Input: part model. Units: mm. Frame: model coordinates. Give positions to 0.01 mm unless a question says otherwise; leave off trailing zeros. Loops run counter-clockwise (first coordinate to the right, second up) from the corner with the lowest first, then second, coordinate; pieces in that order, holes last. Notation, with made-up numbers: (32, 71.5) -> (64, 71.5) arc R8 cw to (64, 83.5) -> close; hole circle Ø8 at (27, 12.5). An arc over 180 degrees is marked (long way). Answer as a JSON object with one key per item and string values. Group by question number.
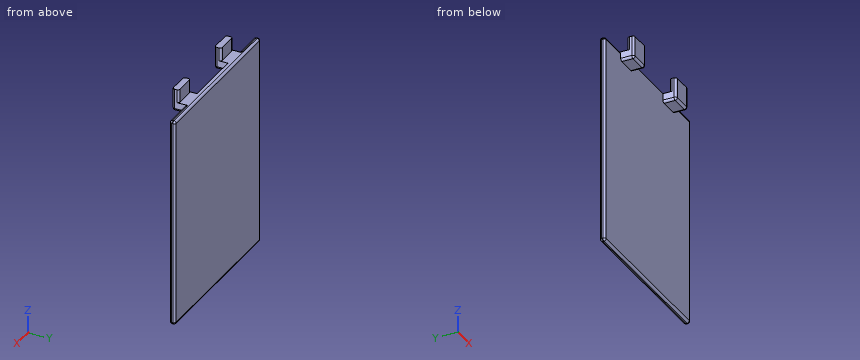
Autodesk Inventor part; units mm, degrees
ref_plane "YZ Plane" through (0, 0, 0) normal (1, 0, 0) x (0, 1, 0)
ref_plane "XZ Plane" through (0, 0, 0) normal (0, 1, 0) x (-1, 0, 0)
ref_plane "XY Plane" through (0, 0, 0) normal (0, 0, 1) x (1, 0, 0)
sketch "Sketch1" plane through (0, 0, 0) normal (0, 1, 0) x (-1, 0, 0)
  line L0 (36.4, 47.4) -> (-36.4, 47.4)
  line L1 (-37.4, 46.4) -> (-37.4, -46.4)
  line L2 (-36.4, -47.4) -> (36.4, -47.4)
  line L3 (37.4, -46.4) -> (37.4, 46.4)
  line L4 (37.4, 47.4) -> (-37.4, -47.4) construction
  line L5 (-37.4, 47.4) -> (37.4, -47.4) construction
  arc A0 (37.4, 46.4) -> (36.4, 47.4) centre (36.4, 46.4) ccw
  arc A1 (-36.4, 47.4) -> (-37.4, 46.4) centre (-36.4, 46.4) ccw
  arc A2 (-37.4, -46.4) -> (-36.4, -47.4) centre (-36.4, -46.4) ccw
  arc A3 (36.4, -47.4) -> (37.4, -46.4) centre (36.4, -46.4) ccw
  point P0 (0, 0)
  dimension "d0" = 94.8
  dimension "d1" = 74.8
  dimension "d2" = 1
extrude "Extrusion1" add sketch "Sketch1" along normal blind 2.5
sketch "Sketch2" plane through (0, 0, 0) normal (0, -1, 0) x (1, 0, 0)
  line L0 (0, 0) -> (-37.4, 0)
  line L1 (-37.4, 0) -> (-37.4, 47.4)
  line L2 (-37.4, 47.4) -> (0, 47.4)
  line L3 (0, 47.4) -> (0, 0)
  line L4 (-23.7, 51.4) -> (-13.7, 51.4)
  line L5 (-13.7, 51.4) -> (-13.7, 43.4)
  line L6 (-13.7, 43.4) -> (-23.7, 43.4)
  line L7 (-23.7, 43.4) -> (-23.7, 51.4)
  line L8 (-36.4, 47.4) -> (36.4, 47.4)
  line L9 (-23.7, 51.4) -> (-13.7, 43.4) construction
  line L10 (-13.7, 51.4) -> (-23.7, 43.4) construction
  line L11 (0, 0) -> (36.5961, 0)
  line L12 (36.5961, 0) -> (36.5961, 47.4)
  line L13 (36.5961, 47.4) -> (0, 47.4)
  line L14 (0, 47.4) -> (0, 0)
  line L15 (13.2981, 51.4) -> (23.2981, 51.4)
  line L16 (23.2981, 51.4) -> (23.2981, 43.4)
  line L17 (23.2981, 43.4) -> (13.2981, 43.4)
  line L18 (13.2981, 43.4) -> (13.2981, 51.4)
  line L19 (13.2981, 51.4) -> (23.2981, 43.4) construction
  line L20 (23.2981, 51.4) -> (13.2981, 43.4) construction
  point P0 (-18.7, 47.4)
  point P1 (18.2981, 47.4)
  point P2 (23.2981, 47.4)
  point P3 (13.2981, 47.4)
  point P4 (-13.7, 47.4)
  point P5 (-23.7, 47.4)
  dimension "d5" = 10
  dimension "d6" = 8
  dimension "d7" = 10
  dimension "d8" = 8
extrude "Extrusion2" add sketch "Sketch2" along normal blind 6 contours L5 L6 L7 L2 | L8 L16 L17 L18
sketch "Sketch3" plane through (-36.4, 2.5, 47.4) normal (0, 0, 1) x (1, 0, 0)
  line L0 (12.7, -8.5) -> (22.7, -8.5)
  line L1 (22.7, -2.5) -> (22.7, -8.5)
  line L2 (13.7, -8.5) -> (21.7, -8.5)
  line L3 (22.7, -7.5) -> (22.7, -6.5)
  line L4 (21.7, -5.5) -> (13.7, -5.5)
  line L5 (12.7, -6.5) -> (12.7, -7.5)
  line L6 (59.6981, -2.5) -> (59.6981, -8.5)
  line L7 (50.6981, -8.5) -> (58.6981, -8.5)
  line L8 (59.6981, -7.5) -> (59.6981, -6.5)
  line L9 (58.6981, -5.5) -> (50.6981, -5.5)
  line L10 (49.6981, -6.5) -> (49.6981, -7.5)
  arc A0 (13.7, -5.5) -> (12.7, -6.5) centre (13.7, -6.5) ccw
  arc A1 (22.7, -6.5) -> (21.7, -5.5) centre (21.7, -6.5) ccw
  arc A2 (21.7, -8.5) -> (22.7, -7.5) centre (21.7, -7.5) ccw
  arc A3 (12.7, -7.5) -> (13.7, -8.5) centre (13.7, -7.5) ccw
  arc A4 (50.6981, -5.5) -> (49.6981, -6.5) centre (50.6981, -6.5) ccw
  arc A5 (59.6981, -6.5) -> (58.6981, -5.5) centre (58.6981, -6.5) ccw
  arc A6 (58.6981, -8.5) -> (59.6981, -7.5) centre (58.6981, -7.5) ccw
  arc A7 (49.6981, -7.5) -> (50.6981, -8.5) centre (50.6981, -7.5) ccw
  line L11 (49.0159, -7.1882) -> (60.5232, -7.1882)
  line L12 (60.5232, -7.1882) -> (60.5232, -9.9786)
  line L13 (60.5232, -9.9786) -> (49.0159, -9.9786)
  line L14 (49.0159, -9.9786) -> (49.0159, -7.1882)
  line L15 (11.7436, -7.1882) -> (24.9599, -7.1882)
  line L16 (24.9599, -7.1882) -> (24.9599, -11.0237)
  line L17 (24.9599, -11.0237) -> (11.7436, -11.0237)
  line L18 (11.7436, -11.0237) -> (11.7436, -7.1882)
  line L19 (49.6981, -8.5) -> (59.6981, -8.5)
  line L20 (49.0159, -8.5834) -> (59.6981, -8.5)
  line L21 (49.6981, -8.5) -> (59.6981, -8.5)
  point P0 (36.4, -2.5)
  point P1 (22.7, -5.5)
  point P2 (59.6981, -5.5)
  point P3 (12.7, -7.1882)
  point P4 (22.7, -7.1882)
  point P5 (49.6981, -7.1882)
  dimension "d11" = 1
extrude "Extrusion3" add sketch "Sketch3" along normal blind 6 contours A3 L5 L15 L1 A2 L0 | L5 A0 L4 A1 L1 L15 | A6 L7 A7 L10 L11 L6 | L11 L10 A4 L9 A5 L6
extrude "Extrusion4" cut sketch "Sketch3" against normal blind 6 contours L0 L1 L15 L16 L17 L18 L5 A3 | A2 L1 L0 | L6 L19 A6 | L20 L14 L11 L10 A7 L7 L19
fillet "Fillet1" radius 1 10 edges at (23.0052, -5.7071, 43.4) (18.2981, -6, 43.4) (13.591, -5.7071, 43.4) (13.2981, -2.5, 43.4) (23.2981, -2.5, 43.4) (-13.9929, -5.7071, 43.4) (-18.7, -6, 43.4) (-23.4071, -5.7071, 43.4) (-23.7, -2.5, 43.4) (-13.7, -2.5, 43.4)
fillet "Fillet2" radius 1 17 edges at (37.1071, 0, -47.1071) (0, 0, -47.4) (-37.1071, 0, -47.1071) (-37.4, 0, 0) (-37.1071, 0, 47.1071) (-30.05, 0, 47.4) (37.1071, 0, 47.1071) (29.849, 0, 47.4) (37.4, 0, 0) (37.1071, 2.5, -47.1071) (0, 2.5, -47.4) (-37.1071, 2.5, -47.1071) (-37.4, 2.5, 0) (-37.1071, 2.5, 47.1071) (0, 2.5, 47.4) (37.1071, 2.5, 47.1071) (37.4, 2.5, 0)
properties part number "tapa decaja 2"
Q1. Ray query, probe 1 along X at (y, z) = (-3.5, 46); probe 2 along Y at (x, z) = (-6, -2.5); probe 3 along Z at (x, y) = (-23.5, 1). Return the intervals inside material, ascending.
Q2. Section B-B on x = -1.5. Return the cut outline in (y, z).
Q3. Section A-A on y = -1.75. Return the cut outline in (x, z), then the cut area to 3 significant figures.
Q4. Section D-D on x = -21. Return the cut outline in (y, z), then the cut area to 3 significant figures.
Q5. Pin query (flat end, axial travel): pin 1 Ø2 at (x, y) = (-21, 0.5) entering from +Z; pin 2 Ø2.5 at (y, z) = (-2, 51) entering from +X; pin 3 Ø3 at (x, y) = (-3, -2.5) entering from +Z; pin 4 Ø3 at (x, z) = (-18.5, 51.5) entering from +Y. Return the tip coordinate at first contact, or that it passes through.
Q6. Section C-C on z = 15. Return the cut outline in (x, y), then the cut area to 3 significant figures.
Numbers:
{
 "1": {"probe 1": "x = -23.7 to -13.7, 13.3 to 23.3", "probe 2": "y = 0 to 2.5", "probe 3": "z = -47.4 to 47.4"},
 "2": {"outline": "(0, -46.4) arc R1 ccw to (1, -47.4) -> (1.5, -47.4) arc R1 ccw to (2.5, -46.4) -> (2.5, 46.4) arc R1 ccw to (1.5, 47.4) -> (0, 47.4) -> close"},
 "3": {"outline": "(-23.7, 44.4) arc R1 ccw to (-22.7, 43.4) -> (-14.7, 43.4) arc R1 ccw to (-13.7, 44.4) -> (-13.7, 47.4) -> (-23.7, 47.4) -> close; (13.3, 44.4) arc R1 ccw to (14.3, 43.4) -> (22.3, 43.4) arc R1 ccw to (23.3, 44.4) -> (23.3, 47.4) -> (13.3, 47.4) -> close", "area": "79.1 mm²"},
 "4": {"outline": "(-6, 44.4) arc R1 ccw to (-5, 43.4) -> (0, 43.4) -> (0, -46.4) arc R1 ccw to (1, -47.4) -> (1.5, -47.4) arc R1 ccw to (2.5, -46.4) -> (2.5, 46.4) arc R1 ccw to (1.5, 47.4) -> (-3, 47.4) -> (-3, 53.4) -> (-6, 53.4) -> close", "area": "278 mm²"},
 "5": {"pin 1": "stops at z = 47.4", "pin 2": "stops at x = 22.96", "pin 3": "passes through", "pin 4": "stops at y = -3"},
 "6": {"outline": "(-37.4, 1) arc R1 ccw to (-36.4, 0) -> (36.4, 0) arc R1 ccw to (37.4, 1) -> (37.4, 1.5) arc R1 ccw to (36.4, 2.5) -> (-36.4, 2.5) arc R1 ccw to (-37.4, 1.5) -> close", "area": "186 mm²"}
}
